Geometry: final body of the model. Coordinates: model frame, mm. Face numbers are marked on the shaded views. Give positions to 0.01 mm unless a question says otherwise; leave off trailing zeros. Loops run counter-clockwise (first coordinate to the right, second up) from the corner with the lowest first, then second, coordinate; pieces in that order, holes last. Notation, with made-up numbers: (52.5, -23) - (63.5, -23) arc R24 ccw to (63.5, 11) - close; hole circle Ø3 at (79.25, 30). An arc over 180 degrees is marked (long way). Answer in a Markdown table with one row per item.
from build123d import *

# Parameters (mm, degrees)
SKETCH1_R           = 10
SKETCH1_R_2         = 1
BOSS_EXTRUDE1_DEPTH = 2
SKETCH2_R           = 3.5
SKETCH2_R_2         = 2.5
BOSS_EXTRUDE2_DEPTH = 5
CUT_EXTRUDE1_REACH  = 17
SKETCH3_R           = 1.25
CIRPATTERN1_COUNT   = 3
SKETCH4_R           = 2.5
SKETCH4_R_2         = 1
BOSS_EXTRUDE3_DEPTH = 3
SKETCH5_R           = 2
CUT_EXTRUDE2_DEPTH  = 4
BOSS_EXTRUDE4_START = -2
BOSS_EXTRUDE4_DEPTH = 2
CIRPATTERN2_COUNT   = 24


with BuildPart() as part:
    # Sketch1 → Boss-Extrude1 (new body)
    with BuildSketch(Plane(origin=(0, 0, 0), x_dir=(1, 0, 0), z_dir=(0, 1, 0))):
        with Locations(Location((0, 0, 0), (0, 0, 270))):
            Circle(SKETCH1_R)
        with Locations(Location((0, 0, 0), (0, 0, 270))):
            Circle(SKETCH1_R_2, mode=Mode.SUBTRACT)
    extrude(amount=BOSS_EXTRUDE1_DEPTH)

    # Sketch2 → Boss-Extrude2 (add)
    with BuildSketch(Plane(origin=(0, 2, 0), x_dir=(1, 0, 0), z_dir=(0, 1, 0))):
        with Locations(Location((0, 0, 0), (0, 0, 270))):
            Circle(SKETCH2_R)
        with Locations(Location((0, 0, 0), (0, 0, 270))):
            Circle(SKETCH2_R_2, mode=Mode.SUBTRACT)
    extrude(amount=BOSS_EXTRUDE2_DEPTH)

    # Sketch3 → Cut-Extrude1 (cut, up to next)
    with BuildSketch(Plane(origin=(0, 2, 0), x_dir=(1, 0, 0), z_dir=(0, 1, 0)), mode=Mode.PRIVATE) as cut_extrude1_sk1:
        with Locations(Location((0, 7.5, 0), (0, 0, 270))):
            Circle(SKETCH3_R)
    cut_extrude1_tool1 = extrude(cut_extrude1_sk1.sketch, amount=-CUT_EXTRUDE1_REACH, mode=Mode.PRIVATE) & part.part
    cut_extrude1 = cut_extrude1_tool1.solids().sort_by_distance((0, 2, -7.5))[0]
    add(cut_extrude1, mode=Mode.SUBTRACT)

    # CirPattern1: Cut-Extrude1 ×3 about axis
    cirpattern1_axis = Axis((0, 0, 0), (0, 1, 0))
    for i in range(1, CIRPATTERN1_COUNT):
        add(cut_extrude1.rotate(cirpattern1_axis, i * 360 / CIRPATTERN1_COUNT), mode=Mode.SUBTRACT)

    # Sketch4 → Boss-Extrude3 (add)
    with BuildSketch(Plane(origin=(0, 2, 0), x_dir=(1, 0, 0), z_dir=(0, 1, 0))):
        with Locations(Location((0, 0, 0), (0, 0, 270))):
            Circle(SKETCH4_R)
        with Locations(Location((0, 0, 0), (0, 0, 270))):
            Circle(SKETCH4_R_2, mode=Mode.SUBTRACT)
    extrude(amount=BOSS_EXTRUDE3_DEPTH)

    # Sketch5 → Cut-Extrude2 (cut)
    with BuildSketch(Plane.XZ):
        with Locations(Location((0, 0, 0), (0, 0, 270))):
            Circle(SKETCH5_R)
    extrude(amount=-CUT_EXTRUDE2_DEPTH, mode=Mode.SUBTRACT)

    # Sketch6 → Boss-Extrude4 (add)
    with BuildSketch(Plane(origin=(0, 7, 0), x_dir=(1, 0, 0), z_dir=(0, 1, 0)).offset(BOSS_EXTRUDE4_START)):
        with BuildLine():
            ThreePointArc((-0.249687304, 2.4875), (0, 2.25), (0.249687304, 2.4875))
            ThreePointArc((0.249687304, 2.4875), (0, 2.5), (-0.249687304, 2.4875))
        make_face()
    boss_extrude4 = extrude(amount=BOSS_EXTRUDE4_DEPTH)

    # CirPattern2: Boss-Extrude4 ×24 about axis
    cirpattern2_axis = Axis((0, 0, 0), (0, 1, 0))
    for i in range(1, CIRPATTERN2_COUNT):
        add(boss_extrude4.rotate(cirpattern2_axis, i * 360 / CIRPATTERN2_COUNT))


solid = part.part
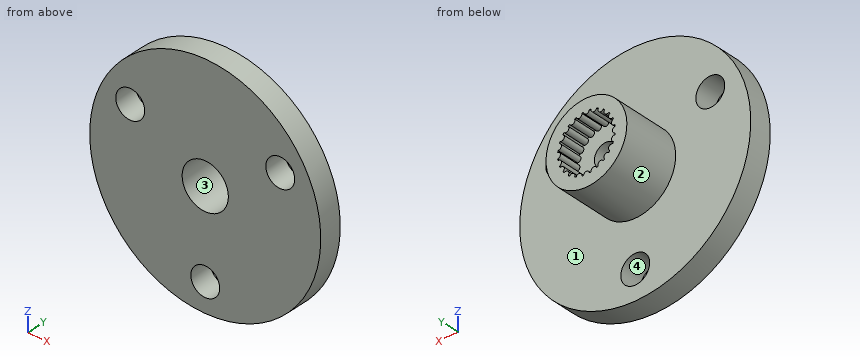
Q1. First-contact query: pin 1 (2 mm diameter, centred on x = -6.5, z = 3.75, fed in from -Y); pin 2 (10 mm diameter, centred on x = -4.5, z = 3.5, fed in from +Y); pin 3 (1.5 mm diameter, centred on x = 0.5, z = -0.5, fed in from +Y); pin 4 (1.5 mm diameter, centred on x = 2.5, y = 3, fed in from -Z). Flat tips, straight axial feed; report the tip coordinate or a pass-through.
Check values:
| item | result |
|---|---|
| pin 1 | through |
| pin 2 | y = 7 |
| pin 3 | y = 5 |
| pin 4 | z = -3.03 |
Q2. Cut plane C-C (x = 7.5). Output: boundary loops of the cut face in (y, z).
Check values:
| item | result |
|---|---|
| outline | (0, -6.61) - (2, -6.61) - (2, 3.01) - (0, 3.01) - close; (0, 4.49) - (2, 4.49) - (2, 6.61) - (0, 6.61) - close |
Q3. Draft query along Z for the marked faces 1, 2, 3 and 4. Return one class per face: pulls with the +Z half, pulls with the -Z half, needs draft (parallel to the pull), parting line crosses it, or undercut.
Check values:
| item | result |
|---|---|
| face 1 | needs draft |
| face 2 | parting line crosses it |
| face 3 | undercut |
| face 4 | undercut |
Q4. Material intervals for line 1 along X through (y, z) = (2.25, 0); line 2 along Y through (x, z) = (-4.25, -0.25); line 3 along Z through (x, y) = (-0.75, 2.5), sorted ascending.
Check values:
| item | result |
|---|---|
| line 1 | -3.5 to -2, 2 to 3.5 |
| line 2 | 0 to 2 |
| line 3 | -3.42 to -1.85, 1.85 to 3.42 |
Q5. Cut plane B-B (x = 0). Output: boundary loops of the cut face in (y, z), and give its area (3 significant figures).
Check values:
| item | result |
|---|---|
| outline | (0, -10) - (2, -10) - (2, -8.75) - (0, -8.75) - close; (0, -6.25) - (2, -6.25) - (2, -3.5) - (7, -3.5) - (7, -2.25) - (5, -2.25) - (5, -1) - (4, -1) - (4, -2) - (0, -2) - close; (0, 2) - (4, 2) - (4, 1) - (5, 1) - (5, 2.25) - (7, 2.25) - (7, 3.5) - (2, 3.5) - (2, 10) - (0, 10) - close |
| area | 43.0 mm² |
Q6. Cut plane D-D (z = 3.75). Output: boundary loops of the cut face in (x, y), and give its area (3 significant figures).
Check values:
| item | result |
|---|---|
| outline | (-9.27, 0) - (-7.75, 0) - (-7.75, 2) - (-9.27, 2) - close; (-5.25, 0) - (5.25, 0) - (5.25, 2) - (-5.25, 2) - close; (7.75, 0) - (9.27, 0) - (9.27, 2) - (7.75, 2) - close |
| area | 27.1 mm² |
Q7. Cut plane A-A (z = 0). Output: boundary loops of the cut face in (x, y), and give its area (3 significant figures).
Check values:
| item | result |
|---|---|
| outline | (-10, 0) - (-2, 0) - (-2, 4) - (-1, 4) - (-1, 5) - (-2.25, 5) - (-2.25, 7) - (-3.5, 7) - (-3.5, 2) - (-10, 2) - close; (1, 4) - (2, 4) - (2, 0) - (10, 0) - (10, 2) - (3.5, 2) - (3.5, 7) - (2.25, 7) - (2.25, 5) - (1, 5) - close |
| area | 48.0 mm² |
